Check sheet for the modelled part. Datum: model origin and axes. Units: mm. Coordinates: 2 decimals unless noted, no trailing zeros. Order: outer loops, then holes, each group sorted by start corner. A loop starts at its lowest first (then second) coordinate and runs counter-clockwise, first axis right, second up.
from build123d import *

# Parameters (mm, degrees)
BOSS_EXTRUDE3_DEPTH       = 3.175
F_8_CLEARANCE_HOLE1_D     = 4.4958
F_8_CLEARANCE_HOLE1_DEPTH = 41.402
F_8_CLEARANCE_HOLE1_TIP   = 1.350674586
F_8_CLEARANCE_HOLE2_D     = 4.4958
F_8_CLEARANCE_HOLE2_DEPTH = 41.402
F_8_CLEARANCE_HOLE2_TIP   = 1.350674586


with BuildPart() as part:
    # Sketch7 → Boss-Extrude3 (new body)
    with BuildSketch(Plane(origin=(0, 0, 0), x_dir=(1, 0, 0), z_dir=(0, 1, 0))):
        with BuildLine():
            Line((5.530913955, 21.842048142), (5.530913955, 7.688957681))
            ThreePointArc((5.530913955, 7.688957681), (5.164609953, 3.502083783), (4.07682791, -0.55757407))
            Line((4.07682791, -0.55757407), (3.77913049, -1.37549101))
            ThreePointArc((3.77913049, -1.37549101), (-0.758308624, -3.949527922), (-4.019818623, 0.121905765))
            Line((-4.019818623, 0.121905765), (-3.35704347, 21.976786093))
            ThreePointArc((-3.35704347, 21.976786093), (1.153290671, 26.286537469), (5.530913955, 21.842048142))
        make_face()
    extrude(amount=BOSS_EXTRUDE3_DEPTH)

    # #8 Clearance Hole1
    with Locations(Plane(origin=(0, 3.175, 0), x_dir=(1, 0, 0), z_dir=(0, 1, 0))):
        with Locations((2.17182791, 5.967048142), (0, 0)):
            Hole(F_8_CLEARANCE_HOLE1_D / 2, depth=F_8_CLEARANCE_HOLE1_DEPTH)
            with Locations((0, 0, -(F_8_CLEARANCE_HOLE1_DEPTH + F_8_CLEARANCE_HOLE1_TIP / 2))):  # 118° drill point
                Cone(0, F_8_CLEARANCE_HOLE1_D / 2, F_8_CLEARANCE_HOLE1_TIP, mode=Mode.SUBTRACT)

    # #8 Clearance Hole2
    with Locations(Plane(origin=(0, 3.175, 0), x_dir=(1, 0, 0), z_dir=(0, 1, 0))):
        with Locations((1.085913955, 21.842048142), (1.085913955, 15.492048142)):
            Hole(F_8_CLEARANCE_HOLE2_D / 2, depth=F_8_CLEARANCE_HOLE2_DEPTH)
            with Locations((0, 0, -(F_8_CLEARANCE_HOLE2_DEPTH + F_8_CLEARANCE_HOLE2_TIP / 2))):  # 118° drill point
                Cone(0, F_8_CLEARANCE_HOLE2_D / 2, F_8_CLEARANCE_HOLE2_TIP, mode=Mode.SUBTRACT)


solid = part.part
(1) Thickness scan on probe 1 along Z at (x, y) = (2.5, 0.9); probe 2 along Z at (x, y) = (-0.75, 1.8); probe 3 along Z at (x, y) = (0.5, 1.05). Record the ranges inside material, lowest first.
Filled in:
probe 1: z = -26.06 to -23.59, -20.09 to -17.24, -13.74 to -8.19, -3.74 to 3.15
probe 2: z = -25.89 to -23.14, -20.54 to -16.79, -14.19 to -2.12, 2.12 to 3.95
probe 3: z = -26.25 to -24.01, -19.67 to -17.66, -13.32 to -7.47, -4.46 to -2.19, 2.19 to 3.99
(2) Go/stop test with flat-tipped pins: P1, Ø4, axis at x = 2.17, z = -5.97, coming from the +Y side; P2, Ø1, axis at x = 3.5, y = 2, coming from the +Z side. Record where each tip stops, or that it passes through.
Filled in:
P1: passes through
P2: stops at z = 2.68
(3) Cross-section at B-B (y = 0.9). Enter the section's corners in (x, z) (1 decimal).
Filled in:
outline: (-4, -0.1) - (-3.4, -22) arc R4.4 ccw to (5.5, -21.8) - (5.5, -7.7) arc R24.1 ccw to (4.1, 0.6) - (3.8, 1.4) arc R4 ccw to start; hole circle Ø4.5 at (0, 0); hole circle Ø4.5 at (1.1, -21.8); hole circle Ø4.5 at (1.1, -15.5); hole circle Ø4.5 at (2.2, -6)
(4) Cross-section at A-A (z = -21). Enter the section's corners in (x, y) (3 decimals), and give its area (3 significant figures).
Filled in:
outline: (-3.387, 0) - (-0.998, 0) - (-0.998, 3.175) - (-3.387, 3.175) - close; (3.17, 0) - (5.531, 0) - (5.531, 3.175) - (3.17, 3.175) - close
area: 15.1 mm2
(5) Release check for a two-part mould opening along Z. For faces 1 (the flat face through (1, 3.175, -11)), 2 (the flat face through (3.93, 1.57, 0.96)), 3 (the cylindrical face through (1.38, 1.57, -24.07)) record: +Z half, -Z half, draft (parallel to the pull), parting line (faces both ways), or undercut.
Filled in:
face 1: draft
face 2: +Z half
face 3: undercut
(6) Cross-section at C-C (x = 3). Enter the section's corners in (y, z) (3 decimals), and give its area (3 significant figures).
Filled in:
outline: (0, -25.854) - (3.175, -25.854) - (3.175, -23.021) - (0, -23.021) - close; (0, -20.663) - (3.175, -20.663) - (3.175, -16.671) - (0, -16.671) - close; (0, -14.313) - (3.175, -14.313) - (3.175, -8.057) - (0, -8.057) - close; (0, -3.877) - (3.175, -3.877) - (3.175, 2.678) - (0, 2.678) - close
area: 62.4 mm2
(7) Cross-section at D-D (z = -5). Enter the section's corners in (x, y) (1 decimal).
Filled in:
outline: (-3.9, 0) - (0.1, 0) - (0.1, 3.2) - (-3.9, 3.2) - close; (4.2, 0) - (5.4, 0) - (5.4, 3.2) - (4.2, 3.2) - close
